Geometry: final body of the model. Coordinates: model frame, mm. A direction names the side the tool comes from. Round coordinates to 2 decimals unless told otherwise and drop trailing zeros. Loops run counter-clockwise (first coordinate to the right, second up) from the corner with the lowest first, then second, coordinate; pieces in that order, holes last. Notation, with made-up numbers: (-15.5, -33) - (38.5, -33) arc R30 ccw to (38.5, -8) - close; hole circle Ø6 at (34, 67.25). An arc over 180 degrees is marked (long way). Answer as a JSON object with one key per item and string values. Group by question number.
Item 1: First-contact query: pin 1 (2 mm diameter, centred on y = 4.5, z = 2, fed in from +X); pin 2 (2 mm diameter, centred on x = 0, y = 3.5, fed in from +Z); pin 3 (0.9 mm diameter, centred on x = 0, y = -1, fed in from +Z). Flat tips, straight axial feed; report the tip coordinate or a pass-through.
Item 2: Section A-A (y = 7.25). Return the cut outline in (x, z).
Item 3: Reachability of faces 4 (the face through (-0.87, -0.95, -0.49)), 5 (the face through (0, 0, 2)) from +Z, -Z, +X, -X, +Y, -Y: full face, straight path, thin tool, end or side. Return the list, or none.
Item 4: Line query: line 1 (X direction, y = 6.25, z = -0.1); line 2 (Z direction, x = 0.75, y = -0.75). Output: solid intervals per line, ascending.
Item 5: Draft query along X for faces 1 (the face through (-1.5, 4, -0.07)), 2 (the face through (0.87, -0.95, 0.49)), 3 (the face through (0, 8, 0)). Return one class per face: released by +X, released by -X, zero draft, split by the parting line, or undercut.
Solid Edge part; units mm, degrees
sketch "Sketch1" plane through (0, 0, 0) normal (0, 0, 1) x (1, 0, 0)
  line L0 (1.5, 0) -> (1.5, 8)
  line L1 (0, 8) -> (1.5, 8)
  line L2 (0, 0) -> (0, 8)
  line L3 (0, 0) -> (0, -1.65)
  line L4 (0, -1.65) -> (2.85, -1.65)
  line L5 (2.85, -1.65) -> (2.85, 0)
  line L6 (2.85, 0) -> (1.5, 0)
revolve "RevolvedProtrusion1" add sketch "Sketch1" angle 360 about axis through (0, 0, 0) along (0, 1, 0)
sketch "Sketch2" plane through (0, 0, 0) normal (1, 0, 0) x (0, 1, 0)
  line L0 (-1.65, 1.6515) -> (-0.61, 1.6515)
  line L1 (0.3435, 0) -> (-0.61, 1.6515)
  line L2 (-1.65, 0) -> (0.3435, 0)
  line L3 (-1.65, 0) -> (-1.65, 1.6515)
revolve "RevolvedCutout1" cut sketch "Sketch2" angle 360 about axis through (0, -4.5, 0) along (0, 1, 0)
sketch "Sketch3" plane through (0, -1.65, 0) normal (0, -1, 0) x (0, 0, 1)
  circle A0 centre (0, 0) radius 1.6515
  line L0 (-1, -0.5774) -> (0, -1.1547)
  line L1 (0, -1.1547) -> (1, -0.5774)
  line L2 (1, -0.5774) -> (1, 0.5774)
  line L3 (1, 0.5774) -> (0, 1.1547)
  line L4 (0, 1.1547) -> (-1, 0.5774)
  line L5 (-1, 0.5774) -> (-1, -0.5774)
extrude "Protrusion1" add sketch "Sketch3" against normal up to next
sketch "Sketch4" plane through (0, 0, 0) normal (0, 0, 1) x (1, 0, 0)
  line L0 (-1.1547, -1.65) -> (0, -1.65)
  line L1 (0, -1.65) -> (0, -1.3406)
  line L2 (0, -1.3406) -> (-1.1547, -1.65)
revolve "RevolvedCutout2" cut sketch "Sketch4" angle 360 about axis through (0, -4.5, 0) along (0, 1, 0)
fillet "Round1" radius 0.1 1 edges at (0, 0, -1.5)
chamfer "倒斜角_2" distance 0.2 angle 45 1 edges at (0, 8, -1.5)
cosmetic_thread "螺纹_3" thread depth 7
sketch "Sketch5" plane through (0, 0, 0) normal (0, 0, 1) x (1, 0, 0)
  arc A0 (-1.5353, -1.65) -> (-2.85, 0) centre (-1.1572, 0) cw
revolve "RevolvedCutout3" cut sketch "Sketch5" angle 360 about axis through (0, 0, 0) along (0, -1, 0) material side at (-2.5202, -1.086, 0)
Values:
{
 "1": {"pin 1": "stops at x = 1.12", "pin 2": "stops at z = 1.5", "pin 3": "stops at z = 2.76"},
 "2": {"outline": "circle Ø3 at (0, 0)"},
 "3": {"face 4": "-Y", "face 5": "+Y"},
 "4": {"line 1": "x = -1.5 to 1.5", "line 2": "z = -2.57 to -0.7, 0.7 to 2.57"},
 "5": {"face 1": "split by the parting line", "face 2": "undercut", "face 3": "zero draft"}
}
